```python
from build123d import *

# Parameters (mm, degrees)
SKETCH2_W          = 15
SKETCH2_H          = 15
CUT_EXTRUDE1_DEPTH = 42.091361623
SKETCH3_R          = 1.5
CUT_EXTRUDE2_DEPTH = 35.372954485


with BuildPart() as part:
    # Sketch1 → Revolve1 (revolve)
    with BuildSketch(Plane.XY, mode=Mode.PRIVATE) as revolve1_sk:
        Polygon((-13, 7.5), (13, 7.5), (13, 13), (12, 13), (12, 22.5), (9, 22.5), (9, 13), (-9, 13), (-9, 22.5), (-12, 22.5), (-12, 13), (-13, 13), align=None)
    revolve(revolve1_sk.sketch.rotate(Axis((0, 0, 0), (1, 0, 0)), 90), axis=Axis((0, 0, 0), (1, 0, 0)))

    # Sketch2 → Cut-Extrude1 (cut, through all)
    with BuildSketch(Plane(origin=(13, 0, 0), x_dir=(0, 0, -1), z_dir=(1, 0, 0))):
        Rectangle(SKETCH2_W, SKETCH2_H)
    extrude(amount=-CUT_EXTRUDE1_DEPTH, mode=Mode.SUBTRACT)

    # Sketch3 → Cut-Extrude2 (cut, through all)
    with BuildSketch(Plane.XY):
        with Locations((7, 0)):
            Circle(SKETCH3_R)
    extrude(amount=-CUT_EXTRUDE2_DEPTH, mode=Mode.SUBTRACT)


solid = part.part
```
CAD build for the part. Positions are in the model's coordinates, mm. A direction names the side the tool comes from. Round coordinates to 2 decimals unless told otherwise and drop trailing zeros. Order: outer loops, then holes, each group sorted by start corner. A loop starts at its lowest first (then second) coordinate and runs counter-clockwise, first axis right, second up. Notation, with made-up numbers: (-35, -4.5) - (-7, -4.5) arc R18 cw to (-7, 21.5) - close; hole circle Ø6 at (-21, 28). An arc over 180 degrees is marked (long way). Answer as CSV lines item,"result". Start each with the question number.
1. Pin check, flat tips, straight feed: pin 1 (4 mm diameter, centred on y = 15, z = 12, fed in from -X); pin 2 (7.5 mm diameter, centred on x = 5, y = 1.5, fed in from -Z); pin 3 (8 mm diameter, centred on x = 6, z = -5, fed in from +Y). Stop position of each tip, or through.
2. Saw through at A-A, the plane z = 0. Write the cut outline in (x, y), and give its area (3 significant figures).
3. Saw through at B-B, the plane y = 0. Write the cut outline in (x, z), and give its area (4 significant figures).
4. Tool access for faces 4 (the face through (5.5, 0.07, -10.21)), 5 (the face through (-12, 10, 10)), 6 (the face through (0, 7.5, 0)), 7 (the face through (-9, 10, -10)): list every direction of +Z, -Z, +X, -X, +Y, -Y with a clear straight run to the whole face (end or side of a thin tool).
5. Saw through at C-C, the plane y = -6.5. Write the cut outline in (x, z).
6. Pull direction Z, two halves, no side cores. Call faces 1 (the face through (0, -7.5, 0)), 2 (the face through (12, 10, -10)), 3 (the face through (-0.1, -3.9, 12.4)): +Z half, -Z half, draft (parallel to the pull), parting line (faces both ways), or undercut.
7. Drill centre lines: L1, parallel to X at y = 0, z = -10.2; L2, parallel to X at y = 2.5, z = -18; L3, parallel to Z at x = -2.5, y = -0.5. Where is each one in solid material? Low to high. Write a range as [from, to].
8. Saw through at D-D, the plane x = 10.75. Write the cut outline in (y, z), and give its area (3 significant figures).
Model answer:
1,pin 1,"stops at x = -12"
1,pin 2,"stops at z = -13"
1,pin 3,"stops at y = 22.38"
2,outline,"(-13, -13) - (-12, -13) - (-12, -22.5) - (-9, -22.5) - (-9, -13) - (9, -13) - (9, -22.5) - (12, -22.5) - (12, -13) - (13, -13) - (13, -7.5) - (-13, -7.5) - close; (-13, 7.5) - (13, 7.5) - (13, 13) - (12, 13) - (12, 22.5) - (9, 22.5) - (9, 13) - (-9, 13) - (-9, 22.5) - (-12, 22.5) - (-12, 13) - (-13, 13) - close"
2,area,"400 mm²"
3,outline,"(-13, -13) - (-12, -13) - (-12, -22.5) - (-9, -22.5) - (-9, -13) - (5.5, -13) - (5.5, -7.5) - (-13, -7.5) - close; (-13, 7.5) - (13, 7.5) - (13, 13) - (12, 13) - (12, 22.5) - (9, 22.5) - (9, 13) - (-9, 13) - (-9, 22.5) - (-12, 22.5) - (-12, 13) - (-13, 13) - close; (8.5, -13) - (9, -13) - (9, -22.5) - (12, -22.5) - (12, -13) - (13, -13) - (13, -7.5) - (8.5, -7.5) - close"
3,area,"383.5 mm²"
4,face 4,"-Z"
4,face 5,"-X"
4,face 6,"+X, -X"
4,face 7,"none"
5,outline,"(-13, -11.26) - (-12, -11.26) - (-12, -21.54) - (-9, -21.54) - (-9, -11.26) - (9, -11.26) - (9, -21.54) - (12, -21.54) - (12, -11.26) - (13, -11.26) - (13, -7.5) - (-13, -7.5) - close; (-13, 7.5) - (13, 7.5) - (13, 11.26) - (12, 11.26) - (12, 21.54) - (9, 21.54) - (9, 11.26) - (-9, 11.26) - (-9, 21.54) - (-12, 21.54) - (-12, 11.26) - (-13, 11.26) - close"
6,face 1,"undercut"
6,face 2,"draft"
6,face 3,"parting line"
7,L1,"x = [-13, 5.5], [8.5, 13]"
7,L2,"x = [-12, -9], [9, 12]"
7,L3,"z = [-12.99, -7.5], [7.5, 12.99]"
8,outline,"circle Ø45 at (0, 0); hole (-7.5, -7.5) - (7.5, -7.5) - (7.5, 7.5) - (-7.5, 7.5) - close"
8,area,"1,370 mm²"
